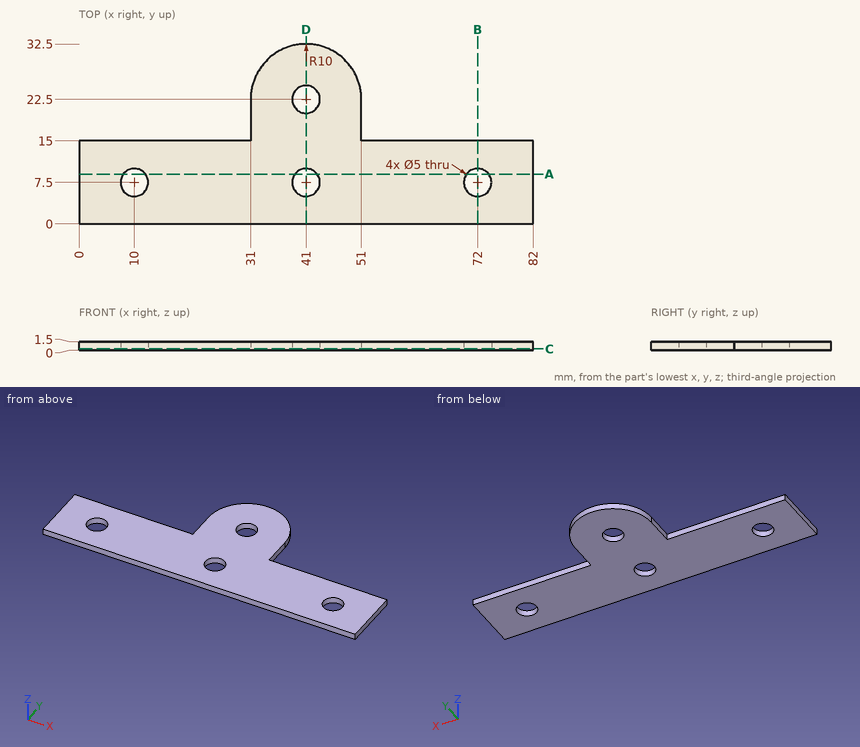
Design review of the part shown in the three views and the two pictorial views. Dimensions are in mm from the part's minimum x, y and z. Coordinates: 2 decimals unless noted, no trailing zeros. Order: outer loops, then holes, each group sorted by start corner. A loop starts at its lowest first (then second) coordinate and runs counter-clockwise, first axis right, second up. Notation, with made-up numbers: (74, 40.25) - (98, 40.25) arc R18 ccw to (98, 69.25) - close; hole circle Ø8 at (4, 3.5). An arc over 180 degrees is marked (long way). Answer as CSV lines item,"result". Start each with the question number.
1) Add section A-A (y = 9). State the section outline as (x, z) points.
2) Add section C-C (z = 0.25). State the section outline as (x, y) points, then the cut area to 3 significant figures.
3) Insertion check: P1, Ø1, axis at x = 29, y = 15, coming from the -Z side; P2, Ø0.8, axis at x = 9, z = 0.5, coming from the +Y side. Each pin has a flat end and moves straight along its axis. Give the tip position at first contact, or say it passes through.
4) To check wall thickness, follow line 1 along Y through (x, z) = (41, 1); line 2 along Y through (x, z) = (72, 0.7); line 3 along Y through (x, z) = (61, 0.6). State the ranges of each line that lie inside material, in increasing order. Write a range as [from, to].
5) Add section D-D (x = 41). State the section outline as (y, z) points, then the cut area to 4 significant figures.
6) Add section B-B (x = 72). State the section outline as (y, z) points, then the cut area to 3 significant figures.
Result:
1,outline,"(0, 0) - (8, 0) - (8, 1.5) - (0, 1.5) - close; (12, 0) - (39, 0) - (39, 1.5) - (12, 1.5) - close; (43, 0) - (70, 0) - (70, 1.5) - (43, 1.5) - close; (74, 0) - (82, 0) - (82, 1.5) - (74, 1.5) - close"
2,outline,"(0, 0) - (82, 0) - (82, 15) - (51, 15) - (51, 22.5) arc R10 ccw to (31, 22.5) - (31, 15) - (0, 15) - close; hole circle Ø5 at (10, 7.5); hole circle Ø5 at (41, 7.5); hole circle Ø5 at (41, 22.5); hole circle Ø5 at (72, 7.5)"
2,area,"1,460 mm^2"
3,P1,"z = 0"
3,P2,"y = 15"
4,line 1,"[0, 5], [10, 20], [25, 32.5]"
4,line 2,"[0, 5], [10, 15]"
4,line 3,"[0, 15]"
5,outline,"(0, 0) - (5, 0) - (5, 1.5) - (0, 1.5) - close; (10, 0) - (20, 0) - (20, 1.5) - (10, 1.5) - close; (25, 0) - (32.5, 0) - (32.5, 1.5) - (25, 1.5) - close"
5,area,"33.75 mm^2"
6,outline,"(0, 0) - (5, 0) - (5, 1.5) - (0, 1.5) - close; (10, 0) - (15, 0) - (15, 1.5) - (10, 1.5) - close"
6,area,"15.0 mm^2"
